from build123d import *

# Parameters (mm, degrees)
SKETCH1_W           = 40
SKETCH1_H           = 25
BOSS_EXTRUDE1_DEPTH = 1
SKETCH2_W           = 40
SKETCH2_H           = 25
BOSS_EXTRUDE2_DEPTH = 1
BOSS_EXTRUDE3_DEPTH = 30
SKETCH5_R           = 1.5
SKETCH5_R_2         = 4
CUT_EXTRUDE2_DEPTH  = 10


with BuildPart() as part:
    # Sketch1 → Boss-Extrude1 (new body)
    with BuildSketch(Plane(origin=(0, 0, 0), x_dir=(0, 0, -1), z_dir=(1, 0, 0))):
        Rectangle(SKETCH1_W, SKETCH1_H)
    extrude(amount=BOSS_EXTRUDE1_DEPTH)

    # Sketch2 → Boss-Extrude2 (add)
    with BuildSketch(Plane(origin=(1, 0, 0), x_dir=(0, 0, -1), z_dir=(1, 0, 0))):
        Rectangle(SKETCH2_W, SKETCH2_H)
    extrude(amount=BOSS_EXTRUDE2_DEPTH)

    # Sketch3 → Boss-Extrude3 (add)
    with BuildSketch(Plane(origin=(2, 0, 0), x_dir=(0, 0, -1), z_dir=(1, 0, 0))):
        Polygon((11.802707793, 1.25), (11.802707793, 3.25), (14.802707793, 3.25), (14.802707793, -3.25), (10.802707793, -3.25), (10.802707793, -1.25), (13, -1.25), (13, 1.25), align=None)
        Polygon((-13, -1.25), (-13, 1.25), (-11.802707793, 1.25), (-11.802707793, 3.25), (-14.802707793, 3.25), (-14.802707793, -3.25), (-10.802707793, -3.25), (-10.802707793, -1.25), align=None)
    extrude(amount=BOSS_EXTRUDE3_DEPTH)

    # Sketch5 → Cut-Extrude2 (cut)
    with BuildSketch(Plane(origin=(2, 0, 0), x_dir=(0, 0, -1), z_dir=(1, 0, 0))):
        with Locations((5, 5)):
            Circle(SKETCH5_R)
        with Locations((5, -5)):
            Circle(SKETCH5_R)
        with Locations((-5, -5)):
            Circle(SKETCH5_R)
        with Locations((-5, 5)):
            Circle(SKETCH5_R)
        Circle(SKETCH5_R_2)
    extrude(amount=-CUT_EXTRUDE2_DEPTH, mode=Mode.SUBTRACT)


solid = part.part
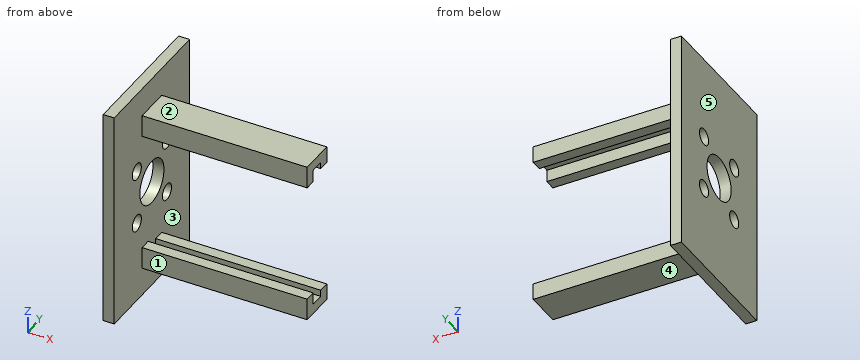
Verification items for the finished model (mm, model axes). Face numbers are marked on the shaded views. A direction names the side the tool comes from. Coordinates: 2 decimals unless noted, no trailing zeros. Order: outer loops, then holes, each group sorted by start corner. A loop starts at its lowest first (then second) coordinate and runs counter-clockwise, first axis right, second up.
1. Go/stop test with flat-tipped pins: pin 1 Ø7.5 at (y, z) = (-3.5, -1) entering from +X; pin 2 Ø1 at (x, z) = (15.5, -12.5) entering from -Y; pin 3 Ø1.5 at (x, z) = (19, -13) entering from +Y; pin 4 Ø7 at (y, z) = (0, 0) entering from -X. Record where each tip stops, or that it passes through.
Results found:
pin 1: stops at x = 2
pin 2: stops at y = -3.25
pin 3: stops at y = 3.25
pin 4: passes through
2. Sectioned sample at B-B, the plane z = -5. Record the cut outline in (x, y).
Results found:
outline: (0, -12.5) - (2, -12.5) - (2, -6.5) - (0, -6.5) - close; (0, -3.5) - (2, -3.5) - (2, 3.5) - (0, 3.5) - close; (0, 6.5) - (2, 6.5) - (2, 12.5) - (0, 12.5) - close
3. Release check for a two-part mould opening along Z. For the marked faces 3, 4 and 5 record: +Z half, -Z half, draft (parallel to the pull), parting line (faces both ways), or undercut.
Results found:
face 3: undercut
face 4: -Z half
face 5: draft
4. Sectioned sample at C-C, the plane x = 16.5. Record the cut outline in (y, z), and give its area (3 significant figures).
Results found:
outline: (-3.25, -14.8) - (3.25, -14.8) - (3.25, -11.8) - (1.25, -11.8) - (1.25, -13) - (-1.25, -13) - (-1.25, -10.8) - (-3.25, -10.8) - close; (-3.25, 10.8) - (-1.25, 10.8) - (-1.25, 13) - (1.25, 13) - (1.25, 11.8) - (3.25, 11.8) - (3.25, 14.8) - (-3.25, 14.8) - close
area: 37.0 mm2
5. Set-up check for the marked faces 1 and 2: record each of +Z, -Z, +X, -X, +Y, -Y from which the full face is reachable in a straight line by a thin tool's end or side.
Results found:
face 1: +Z, -Z, +X, -Y
face 2: +Z, +X, +Y, -Y
6. Scan lines: line 1 (Y direction, x = 1.55, z = 5); line 2 (Y direction, x = 0.5, z = 0); line 3 (Y direction, x = 18.5, z = -12.5). Record each from-to range of solid material in increasing order.
Results found:
line 1: y = -12.5 to -6.5, -3.5 to 3.5, 6.5 to 12.5
line 2: y = -12.5 to -4, 4 to 12.5
line 3: y = -3.25 to -1.25, 1.25 to 3.25
7. Sectioned sample at A-A, the plane y = -5. Record the cut outline in (x, z).
Results found:
outline: (0, -20) - (2, -20) - (2, -6.5) - (0, -6.5) - close; (0, -3.5) - (2, -3.5) - (2, 3.5) - (0, 3.5) - close; (0, 6.5) - (2, 6.5) - (2, 20) - (0, 20) - close
8. Sectioned sample at D-D, the plane y = 0. Record the cut outline in (x, z).
Results found:
outline: (0, -20) - (2, -20) - (2, -14.8) - (32, -14.8) - (32, -13) - (2, -13) - (2, -4) - (0, -4) - close; (0, 4) - (2, 4) - (2, 13) - (32, 13) - (32, 14.8) - (2, 14.8) - (2, 20) - (0, 20) - close
